Can you work these out from the model? Positions are in its coordinate system, mm. Face numbers are marked on the shaded views. A direction names the side the tool comes from. Give positions to 0.01 mm unless a question says otherwise; leave off trailing zeros. Write each loop counter-clockwise with the first axis right and the second up, starting at its lowest first coordinate (ties: lowest second). Pieces come first, ordered by that corner, then holes. Notation, with made-up numbers: M 9.5,-6.75 L 46.5,-6.75 A18 cw 46.5,18.25 Z; hole C -39.75,36.5 d9. An arc over 180 degrees is marked long. Write each question's results on one line, items separated by ' | '.
from build123d import *

# Parameters (mm, degrees)
F0_R     = 28.956
F0_R_2   = 26.67
F1_DEPTH = 31.75
F2_R     = 28.829682
F3_DEPTH = 2.54
F4_R     = 22.625614
F4_R_2   = 17.907
F5_DEPTH = 17.78
F6_R     = 17.965029
F7_DEPTH = 2.54


with BuildPart() as f1:
    # F0 (on Right) → F1 (new body)
    with BuildSketch(Plane.YZ):
        Circle(F0_R)
        Circle(F0_R_2, mode=Mode.SUBTRACT)
    extrude(amount=F1_DEPTH)

    # F2 (on face) → F3 (join)
    with BuildSketch(Plane.YZ.offset(31.75)):
        Circle(F2_R)
    extrude(amount=F3_DEPTH)

    # F4 (on face) → F5 (join)
    with BuildSketch(Plane.YZ.offset(34.29)):
        Circle(F4_R)
        Circle(F4_R_2, mode=Mode.SUBTRACT)
    extrude(amount=F5_DEPTH)

    # F6 (on face) → F7 (cut, through all)
    with BuildSketch(Plane.YZ.offset(34.29)):
        Circle(F6_R)
    extrude(amount=-F7_DEPTH, mode=Mode.SUBTRACT)


solid = f1.part
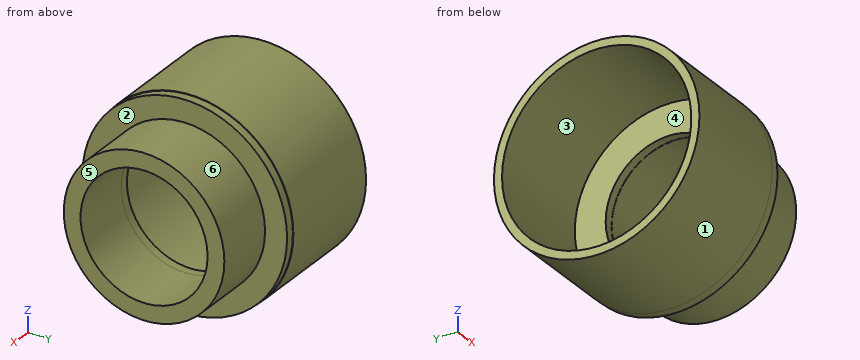
Item 1: Thinking about a two-plate mould opening in Z: for the marked faces 1, 2 and 3, which applies, +Z half, -Z half, draft (parallel to the pull), parting line (faces both ways), or undercut?
Geometry says:
face 1: parting line | face 2: draft | face 3: undercut
Item 2: I'm going to push flat-ended pins straight in: pin 1 (5 mm diameter, centred on x = 36, y = -10, fed in from +Z); pin 2 (17.5 mm diameter, centred on y = -0.5, z = -5.5, fed in from +X); pin 3 (1 mm diameter, centred on x = 22.5, y = 12.5, fed in from -Z); pin 4 (1 mm diameter, centred on y = -14, z = -14, fed in from -X). Where does each tip first touch, or does it pass through?
Geometry says:
pin 1: stops at z = 27.65 | pin 2: passes through | pin 3: stops at z = -26.35 | pin 4: stops at x = 31.75
Item 3: For the marked faces 4, 5 and 6, which set-ups out of +Z, -Z, +X, -X, +Y, -Y let a thin tool reach every point of the face, with its end or its side?
Geometry says:
face 4: -X | face 5: +Z, -Z, +X, +Y, -Y | face 6: +X
Item 4: If I drill on line 1 (Z direction, x = 44, y = 0); line 2 (X direction, y = -20.5, z = 11); line 3 (Z direction, x = 37, y = 10), over which ranges is the centre line in solid material (lowest first)? Write a range as from..to.
Geometry says:
line 1: z = -22.63..-17.91, 17.91..22.63 | line 2: x = 31.75..34.29 | line 3: z = -20.3..-14.85, 14.85..20.3
Item 5: I want a section at C-C, the plane x = 21.5. Please give me the cut outline in (y, z), and give its area (3 significant figures).
Geometry says:
outline: C 0,0 d57.91; hole C 0,0 d53.34 | area: 399 mm2
Item 6: I want a section at A-A, the plane y = -3. Please give me the cut outline in (x, z).
Geometry says:
outline: M 0,-28.8 L 31.75,-28.8 L 31.75,-28.67 L 34.29,-28.67 L 34.29,-22.43 L 52.07,-22.43 L 52.07,-17.65 L 34.29,-17.65 L 34.29,-17.71 L 31.75,-17.71 L 31.75,-26.5 L 0,-26.5 Z; M 0,26.5 L 31.75,26.5 L 31.75,17.71 L 34.29,17.71 L 34.29,17.65 L 52.07,17.65 L 52.07,22.43 L 34.29,22.43 L 34.29,28.67 L 31.75,28.67 L 31.75,28.8 L 0,28.8 Z
Item 7: I want a section at B-B, the plane z = 0. Please give me the cut outline in (x, y).
Geometry says:
outline: M 0,-28.96 L 31.75,-28.96 L 31.75,-28.83 L 34.29,-28.83 L 34.29,-22.63 L 52.07,-22.63 L 52.07,-17.91 L 34.29,-17.91 L 34.29,-17.97 L 31.75,-17.97 L 31.75,-26.67 L 0,-26.67 Z; M 0,26.67 L 31.75,26.67 L 31.75,17.97 L 34.29,17.97 L 34.29,17.91 L 52.07,17.91 L 52.07,22.63 L 34.29,22.63 L 34.29,28.83 L 31.75,28.83 L 31.75,28.96 L 0,28.96 Z
Item 8: I want a section at D-D, the plane y = 19. Please give me the cut outline in (x, z).
Geometry says:
outline: M 0,-21.85 L 31.75,-21.85 L 31.75,-21.68 L 34.29,-21.68 L 34.29,-12.28 L 52.07,-12.28 L 52.07,12.28 L 34.29,12.28 L 34.29,21.68 L 31.75,21.68 L 31.75,21.85 L 0,21.85 L 0,18.72 L 31.75,18.72 L 31.75,-18.72 L 0,-18.72 Z
